The model under review builds one solid part; all positions refer to its coordinate system, in mm. Face numbers are marked on the shaded views. Coordinates: 2 decimals unless noted, no trailing zeros. Order: outer loops, then holes, each group sorted by start corner. A loop starts at its lowest first (then second) coordinate and runs counter-clockwise, first axis right, second up. Notation, with made-up numbers: (-28.75, 52.25) -> (6.25, 52.25) arc R14 cw to (6.25, 58.25) -> close; hole circle Ø1 at (86, 83). An arc over 180 degrees is marked (long way). Put each result on its own line as item: value.
from build123d import *

# Parameters (mm, degrees)
SKETCH1_R     = 4.188
BASENUT_DEPTH = 9.5


with BuildPart() as part:
    # Sketch1 → BaseNut (new body)
    with BuildSketch(Plane.XY):
        Polygon((4.618802154, -8), (9.237604307, 0), (4.618802154, 8), (-4.618802154, 8), (-9.237604307, 0), (-4.618802154, -8), align=None)
        Circle(SKETCH1_R, mode=Mode.SUBTRACT)
    extrude(amount=-BASENUT_DEPTH)

    # Sketch2 → Double-Chamfer (revolve, cut)
    with BuildSketch(Plane(origin=(0, 0, 0), x_dir=(1, 0, 0), z_dir=(0, 1, 0))):
        Polygon((-9.237604307, 9.5), (-7.625, 9.5), (-9.237604307, 8.568962469), align=None)
        Polygon((-9.237604307, 0.931037531), (-9.237604307, 0), (-7.625, 0), align=None)
    revolve(axis=Axis((0, 0, -3.375940562), (0, 0, 1)), mode=Mode.SUBTRACT)


solid = part.part
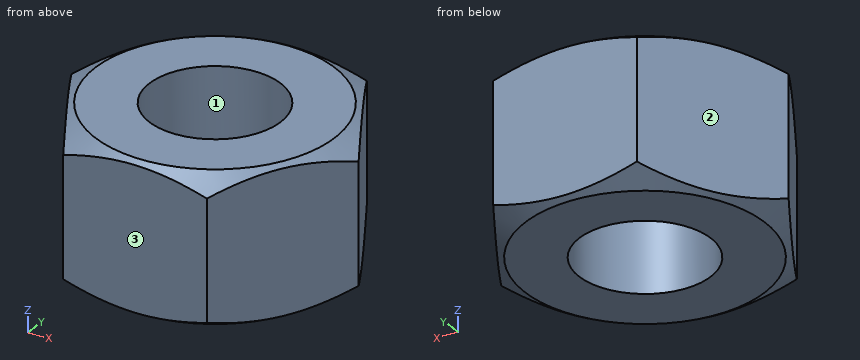
Item 1: Consider section A-A on x = 0. Write out the cut boundary in (y, z) (1 decimal).
Answers below:
outline: (-8, -9.3) -> (-7.6, -9.5) -> (-4.2, -9.5) -> (-4.2, 0) -> (-7.6, 0) -> (-8, -0.2) -> close; (4.2, -9.5) -> (7.6, -9.5) -> (8, -9.3) -> (8, -0.2) -> (7.6, 0) -> (4.2, 0) -> close
Item 2: Consider section C-C on z = -0.5. Write out the cut boundary in (x, y), and give its area (3 significant figures).
Answers below:
outline: (-8.35, -1.54) -> (-5.51, -6.46) arc R8.49 ccw to (-2.85, -8) -> (2.85, -8) arc R8.49 ccw to (5.51, -6.46) -> (8.35, -1.54) arc R8.49 ccw to (8.35, 1.54) -> (5.51, 6.46) arc R8.49 ccw to (2.85, 8) -> (-2.85, 8) arc R8.49 ccw to (-5.51, 6.46) -> (-8.35, 1.54) arc R8.49 ccw to start; hole circle Ø8.38 at (0, 0)
area: 160 mm^2
Item 3: Mouldability with a two-part tool opening along X and no side actions: class the marked faces 1, 2 and 3 as +X half, -X half, draft (parallel to the pull), parting line (faces both ways), or undercut.
Answers below:
face 1: undercut
face 2: -X half
face 3: draft
Item 4: For pin 1 Ø1 at (x, z) = (7.5, -3) entering from +Y, flat-tipped, find the tip position at first contact; note if it passes through.
Answers below:
pin 1: y = 3.88
Item 5: Consider section B-B on z = -7.5. Write out the cut boundary in (x, y), and give its area (3 significant figures).
Answers below:
outline: (-9.24, 0) -> (-4.62, -8) -> (4.62, -8) -> (9.24, 0) -> (4.62, 8) -> (-4.62, 8) -> close; hole circle Ø8.38 at (0, 0)
area: 167 mm^2
Item 6: For line 1 (Y direction, x = 0, z = -3); line 2 (X direction, y = -2.25, z = -8); line 3 (X direction, y = -2.75, z = -6.75), list the stretches that pass through material, from the lowest coordinate up. Write a range as from..to.
Answers below:
line 1: -8..-4.19, 4.19..8
line 2: -7.94..-3.53, 3.53..7.94
line 3: -7.65..-3.16, 3.16..7.65
